```python
from build123d import *
from OCP.BRepFilletAPI import BRepFilletAPI_MakeChamfer

# Parameters (mm, degrees)
SKIZZE1_W                       = 67
SKIZZE1_H                       = 79
SKIZZE1_W_2                     = 40.55
SKIZZE1_H_2                     = 77
AUFSATZ_LINEAR_AUSTRAGEN2_DEPTH = 40
FASE1_SIZE                      = 20.5
FASE1_SIZE2                     = 0.8
VERRUNDUNG2_R                   = 5


with BuildPart() as part:
    # Skizze1 → Aufsatz-Linear austragen2 (new body)
    with BuildSketch(Plane(origin=(0, 0, 0), x_dir=(1, 0, 0), z_dir=(0, 1, 0))):
        with Locations((32.5, 38.5)):
            Rectangle(SKIZZE1_W, SKIZZE1_H)
        with Locations((20.275, 38.5)):
            Rectangle(SKIZZE1_W_2, SKIZZE1_H_2, mode=Mode.SUBTRACT)
    extrude(amount=AUFSATZ_LINEAR_AUSTRAGEN2_DEPTH)

    # Fase1: one chamfer whose edges measure the first distance from different faces: ONE call of the kernel's chamfer builder (chamfer() names one face for all edges)
    fase1_edges_1 = [part.edges().sort_by_distance(p)[0] for p in [
        (66, 40, -38.5),
    ]]
    fase1_side_1 = [part.faces().sort_by_distance(p)[0] for p in [
        (66, 20, -38.5),
    ]]
    fase1_edges_2 = [part.edges().sort_by_distance(p)[0] for p in [
        (32.5, 40, -78),
    ]]
    fase1_side_2 = [part.faces().sort_by_distance(p)[0] for p in [
        (32.5, 20, -78),
    ]]
    fase1_edges_3 = [part.edges().sort_by_distance(p)[0] for p in [
        (-1, 40, -38.5),
    ]]
    fase1_side_3 = [part.faces().sort_by_distance(p)[0] for p in [
        (-1, 20, -38.5),
    ]]
    fase1_edges_4 = [part.edges().sort_by_distance(p)[0] for p in [
        (32.5, 40, 1),
    ]]
    fase1_side_4 = [part.faces().sort_by_distance(p)[0] for p in [
        (32.5, 20, 1),
    ]]
    fase1 = BRepFilletAPI_MakeChamfer(part.part.solid().wrapped)
    for e in fase1_edges_1:
        fase1.Add(FASE1_SIZE, FASE1_SIZE2, e.wrapped, fase1_side_1[0].wrapped)  # the first distance lies on this face
    for e in fase1_edges_2:
        fase1.Add(FASE1_SIZE, FASE1_SIZE2, e.wrapped, fase1_side_2[0].wrapped)  # the first distance lies on this face
    for e in fase1_edges_3:
        fase1.Add(FASE1_SIZE, FASE1_SIZE2, e.wrapped, fase1_side_3[0].wrapped)  # the first distance lies on this face
    for e in fase1_edges_4:
        fase1.Add(FASE1_SIZE, FASE1_SIZE2, e.wrapped, fase1_side_4[0].wrapped)  # the first distance lies on this face
    add(Compound.cast(fase1.Shape()), mode=Mode.REPLACE)

    # Verrundung2
    # the kernel refuses this fillet: 5 mm, written as the material it takes off along each edge
    with BuildSketch(Plane(origin=(-1.24380965, 19.5, -78), x_dir=(0, -1, 0), z_dir=(1, 0, 0)), Plane(origin=(66.24380965, 19.5, 1), x_dir=(0, -1, 0), z_dir=(-1, 0, 0))) as verrundung2_piece_1:
        with BuildLine():
            CenterArc((VERRUNDUNG2_R * 0.019504771978, -VERRUNDUNG2_R), VERRUNDUNG2_R, 90, 2.234798859)
            Line((-VERRUNDUNG2_R * 0.0194899369818, -VERRUNDUNG2_R * 0.000760582906605), (0, 0))
            Line((0, 0), (VERRUNDUNG2_R * 0.019504771978, 0))
        make_face()
    extrude(amount=67.487619299, mode=Mode.SUBTRACT)
    with BuildSketch(Plane(origin=(66, 19.5, -78.24380965), x_dir=(0, -1, 0), z_dir=(0, 0, 1)), Plane(origin=(-1, 19.5, 1.24380965), x_dir=(0, -1, 0), z_dir=(0, 0, -1))) as verrundung2_piece_2:
        with BuildLine():
            CenterArc((VERRUNDUNG2_R * 0.019504771978, -VERRUNDUNG2_R), VERRUNDUNG2_R, 90, 2.234798859)
            Line((-VERRUNDUNG2_R * 0.0194899369818, -VERRUNDUNG2_R * 0.000760582906605), (0, 0))
            Line((0, 0), (VERRUNDUNG2_R * 0.019504771978, 0))
        make_face()
    extrude(amount=79.487619299, mode=Mode.SUBTRACT)


solid = part.part
```
Source: CAD feature listing. Evaluate the final solid. Frame: model axes, mm. A direction names the side the tool comes from. Give positions to 0.01 mm unless a question says otherwise; leave off trailing zeros. Loops run counter-clockwise (first coordinate to the right, second up) from the corner with the lowest first, then second, coordinate; pieces in that order, holes last. Notation, with made-up numbers: (-15.75, 71) -> (41.25, 71) arc R32 cw to (41.25, 110) -> close; hole circle Ø6 at (61.5, 26.25). An arc over 180 degrees is marked (long way). Put each result on its own line as item: value. Start each with the question number.
1) Cut plane D-D (y = 31). Return loops of the section in (x, z).
2) Cut plane B-B (z = -44). Return loops of the section in (x, y), then the cut area to 3 significant figures.
3) Cut plane A-A (y = 12.5). Return loops of the section in (x, z).
4) Material intervals for probe 1 along Z at (x, y) = (36.5, 5); probe 2 along X at (y, z) = (7, -38.5); probe 3 along X at (y, z) = (23, -41.5), sorted ascending.
5) Reachability of faces 5 (the face through (20, 20, 0)), 6 (the face through (66, 10, -38)) from +Z, -Z, +X, -X, +Y, -Y: full face, straight path, thin tool, end or side. Return the list, or none.
6) Cut plane C-C (x = 17). Return loops of the section in (y, z), then the cut area to 3 significant figures.
7) Draft query along Z for faces 1 (the face through (32, 10, 1)), 2 (the face through (32.031, 29.942, -77.593)), 3 (the face through (-0.593, 29.942, -37.947)), 4 (the face through (0, 20, -38)). Return one class per face: released by +Z, released by -Z, zero draft, split by the parting line, or undercut.
8) Contact query for flat-ended pins moving along their axis: P1, Ø6, axis at x = 36, z = -44, coming from the -Y side; P2, Ø1.5, axis at x = 57.5, y = 35, coming from the -Z side; P3, Ø5, axis at x = 53.5, y = 33.5, coming from the -Z side; P4, Ø6, axis at y = 31.5, z = -17, coming from the -X side. Output: stop coordinate, or through.
Results are:
1. outline: (-0.55, -77.55) -> (65.55, -77.55) -> (65.55, 0.55) -> (-0.55, 0.55) -> close; hole (0, -77) -> (40.55, -77) -> (40.55, 0) -> (0, 0) -> close
2. outline: (-1, 0) -> (0, 0) -> (0, 40) -> (-0.2, 40) -> (-1, 19.6) arc R5 ccw to (-1, 19.4) -> close; (40.55, 0) -> (66, 0) -> (66, 19.4) arc R5 ccw to (66, 19.6) -> (65.2, 40) -> (40.55, 40) -> close
2. area: 1,040 mm2
3. outline: (-1, -78) -> (66, -78) -> (66, 1) -> (-1, 1) -> close; hole (0, -77) -> (40.55, -77) -> (40.55, 0) -> (0, 0) -> close
4. probe 1: z = -78 to -77, 0 to 1
4. probe 2: x = -1 to 0, 40.55 to 66
4. probe 3: x = -0.86 to 0, 40.55 to 65.86
5. face 5: +Y, -Y
5. face 6: +Z, -Z, +X, +Y, -Y
6. outline: (0, -78) -> (19.4, -78) arc R5 ccw to (19.6, -78) -> (40, -77.2) -> (40, -77) -> (0, -77) -> close; (0, 0) -> (40, 0) -> (40, 0.2) -> (19.6, 1) arc R5 ccw to (19.4, 1) -> (0, 1) -> close
6. area: 63.6 mm2
7. face 1: released by +Z
7. face 2: released by -Z
7. face 3: zero draft
7. face 4: undercut
8. P1: passes through
8. P2: stops at z = -77.42
8. P3: stops at z = -77.55
8. P4: stops at x = -0.65
